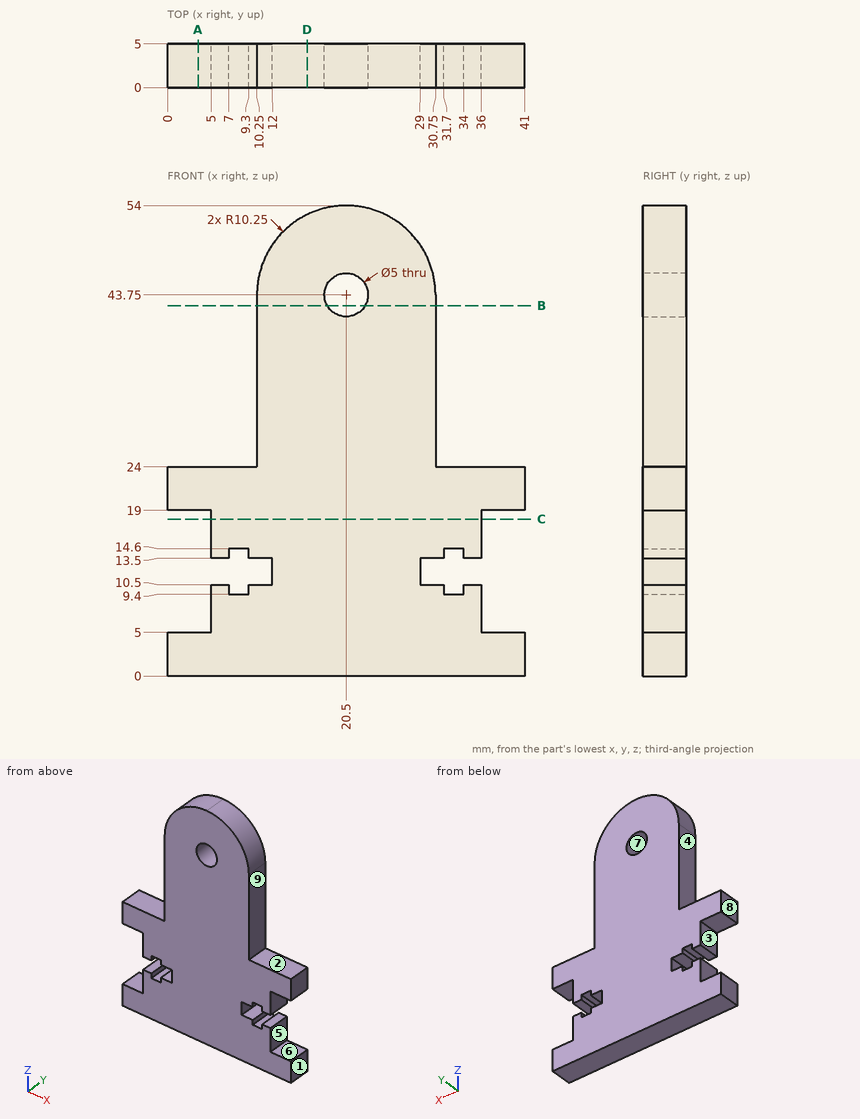
Can you work these out from the drawing? Everything is in mm from the part's minimum corner. A direction names the side the tool comes from. Coordinates: 2 decimals unless noted, no trailing zeros. Loops run counter-clockwise (first coordinate to the right, second up) from the corner with the lowest first, then second, coordinate; pieces in that order, holes last. Notation, with made-up numbers: (68.5, -29) - (107.5, -29) arc R28 ccw to (107.5, -9) - close; hole circle Ø7 at (65, 75). An arc over 180 degrees is marked (long way). Put each result on its own line as item: value. Start each with the question number.
Item 1: For pin 1 (0.9 mm diameter, centred on y = 3, z = 14, fed in from -X); pin 2 (1.5 mm diameter, centred on y = 3.5, z = 11.5, fed in from -X); pin 3 (0.9 mm diameter, centred on y = 3.5, z = 14, fed in from +X), each with a flat end and sliding along its axis, tell me the tip position at first contact or that it passes through.
Item 2: Suppose I cut it at A-A (x = 3.5). Please give me the cut outline in (y, z).
Item 3: If I drill on line 1 along Z through (x, y) = (37.5, 4.35); line 2 along Z through (x, y) = (20.5, 0.3); line 3 along X through (y, z) = (2.25, 43.75), over which ranges is the centre line in solid material (lowest first)?
Item 4: Suppose I cut it at D-D (x = 16). Please give me the cut outline in (y, z), and give its area (3 significant figures).
Item 5: Suppose I cut it at B-B (z = 42.5). Please give me the cut outline in (x, y) (3 decimals).
Item 6: Suppose I cut it at C-C (z = 18). Please give me the cut outline in (x, y).
Item 7: Which directions (+Z, -Z, +X, -X, +Y, -Y) give clear straight access to the entire face, cutting with the end or side of a thin tool? Please do the marked faces 1, 2, 3, 4 and 5.
Item 8: If we mould it in two halves opening along X, with no side actions, what happens to the marked faces 6, 7, 8 and 9? For each: +X half, -X half, draft (parallel to the pull), parting line (faces both ways), or undercut.
Here are the results:
1. pin 1: x = 5
1. pin 2: x = 12
1. pin 3: x = 36
2. outline: (0, 0) - (5, 0) - (5, 5) - (0, 5) - close; (0, 19) - (5, 19) - (5, 24) - (0, 24) - close
3. line 1: 0 to 5, 19 to 24
3. line 2: 0 to 41.25, 46.25 to 54
3. line 3: 10.25 to 18, 23 to 30.75
4. outline: (0, 0) - (5, 0) - (5, 52.96) - (0, 52.96) - close
4. area: 265 mm²
5. outline: (10.25, 0) - (18.335, 0) - (18.335, 5) - (10.25, 5) - close; (22.665, 0) - (30.75, 0) - (30.75, 5) - (22.665, 5) - close
6. outline: (5, 0) - (36, 0) - (36, 5) - (5, 5) - close
7. face 1: +Z, -Z, +X, +Y, -Y
7. face 2: +Z, +X, +Y, -Y
7. face 3: -X, +Y, -Y
7. face 4: +Z, -X, +Y, -Y
7. face 5: +X, +Y, -Y
8. face 6: draft
8. face 7: undercut
8. face 8: -X half
8. face 9: +X half
